```python
from build123d import *

# Parameters (mm, degrees)
IZIM1_R                     = 22.5
Y_KSEKLIK_EKSTR_ZYON1_DEPTH = 32.5
IZIM2_R                     = 17.8
Y_KSEKLIK_EKSTR_ZYON2_DEPTH = 2
RADYUS1_R                   = 0.5
IZIM3_R                     = 13.6
Y_KSEKLIK_EKSTR_ZYON3_DEPTH = 5
RADYUS2_R                   = 2
IZIM4_R                     = 9.05
KES_EKSTR_ZYON1_DEPTH       = 20
RADYUS3_R                   = 0.5
IZIM5_R                     = 18
Y_KSEKLIK_EKSTR_ZYON4_DEPTH = 10.7
IZIM6_R                     = 22.65
Y_KSEKLIK_EKSTR_ZYON5_DEPTH = 5
IZIM7_W                     = 16
IZIM7_H                     = 16
IZIM7_W_2                   = 13
IZIM7_H_2                   = 13
Y_KSEKLIK_EKSTR_ZYON6_DEPTH = 4


with BuildPart() as part:
    # Çizim1 → Yükseklik-Ekstrüzyon1 (new body)
    with BuildSketch(Plane.XY):
        Circle(IZIM1_R)
    extrude(amount=Y_KSEKLIK_EKSTR_ZYON1_DEPTH)

    # Çizim2 → Yükseklik-Ekstrüzyon2 (add)
    with BuildSketch(Plane.XY.offset(32.5)):
        Circle(IZIM2_R)
    extrude(amount=Y_KSEKLIK_EKSTR_ZYON2_DEPTH)

    # Radyus1
    radyus1_edges = [part.edges().sort_by_distance(p)[0] for p in [
        (-17.8, 0, 32.5),
    ]]
    fillet(radyus1_edges, radius=RADYUS1_R)

    # Çizim3 → Yükseklik-Ekstrüzyon3 (add)
    with BuildSketch(Plane.XY.offset(34.5)):
        Circle(IZIM3_R)
    extrude(amount=Y_KSEKLIK_EKSTR_ZYON3_DEPTH)

    # Radyus2
    radyus2_edges = [part.edges().sort_by_distance(p)[0] for p in [
        (-13.6, 0, 34.5),
    ]]
    fillet(radyus2_edges, radius=RADYUS2_R)

    # Çizim4 → Kes-Ekstrüzyon1 (cut)
    with BuildSketch(Plane.XY.offset(39.5)):
        Circle(IZIM4_R)
    extrude(amount=-KES_EKSTR_ZYON1_DEPTH, mode=Mode.SUBTRACT)

    # Radyus3
    radyus3_edges = [part.edges().sort_by_distance(p)[0] for p in [
        (-22.5, 0, 32.5),
    ]]
    fillet(radyus3_edges, radius=RADYUS3_R)

    # Çizim5 → Yükseklik-Ekstrüzyon4 (add)
    with BuildSketch(Plane(origin=(0, 0, 0), x_dir=(-1, 0, 0), z_dir=(0, 0, -1))):
        Circle(IZIM5_R)
    extrude(amount=Y_KSEKLIK_EKSTR_ZYON4_DEPTH)

    # Çizim6 → Yükseklik-Ekstrüzyon5 (add)
    with BuildSketch(Plane(origin=(0, 0, -10.7), x_dir=(-1, 0, 0), z_dir=(0, 0, -1))):
        Circle(IZIM6_R)
    extrude(amount=Y_KSEKLIK_EKSTR_ZYON5_DEPTH)

    # Çizim7 → Yükseklik-Ekstrüzyon6 (add)
    with BuildSketch(Plane(origin=(0, 0, -15.7), x_dir=(-1, 0, 0), z_dir=(0, 0, -1))):
        Rectangle(IZIM7_W, IZIM7_H)
        Rectangle(IZIM7_W_2, IZIM7_H_2, mode=Mode.SUBTRACT)
    extrude(amount=Y_KSEKLIK_EKSTR_ZYON6_DEPTH)


solid = part.part
```
The model under review builds one solid part; all positions refer to its coordinate system, in mm. A direction names the side the tool comes from. Give positions to 0.01 mm unless a question says otherwise; leave off trailing zeros. Write each loop counter-clockwise with the first axis right and the second up, starting at its lowest first coordinate (ties: lowest second). Pieces come first, ordered by that corner, then holes. Notation, with made-up numbers: (-22, -40) -> (-7, -40) arc R34 cw to (-7, -2) -> close; hole circle Ø7 at (-21, 6). An arc over 180 degrees is marked (long way). Answer in a Markdown table with one row per item.
1) Clearance check with flat-ended pins moving along their axes: P1, Ø3, axis at x = -2, z = -17, coming from the -Y side; P2, Ø21, axis at x = 0, y = 0, coming from the +Z side; P3, Ø3, axis at y = -9, z = -4.5, coming from the -X side; P4, Ø4, axis at x = -2, y = -2, coming from the -Z side. State where each tip first meets the part, or that it passes through.
Worked answers:
| item | result |
|---|---|
| P1 | y = -22.62 |
| P2 | z = 39.5 |
| P3 | x = -16.36 |
| P4 | z = -15.7 |
2) Mouldability with a two-part tool opening along Y and no side actions: class faces 1 (the flat face through (-18, -5, 32.5)), 2 (the cylindrical face through (-2.948, -13.277, 37.979)), 3 (the flat face through (6.5, 0, -18)) as +Y half, -Y half, draft (parallel to the pull), parting line (faces both ways), or undercut.
Worked answers:
| item | result |
|---|---|
| face 1 | draft |
| face 2 | parting line |
| face 3 | undercut |
3) For L1, parallel to Z at x = 7, y = 17.5; L2, parallel to Y at x = 0, z = 34; L3, parallel to Y at x = 0, z = 30.25, list the stretches that pass through material, from the lowest coordinate up. Write a range as [from, to].
Worked answers:
| item | result |
|---|---|
| L1 | [-15.7, -10.7], [0, 32.5] |
| L2 | [-17.8, -9.05], [9.05, 17.8] |
| L3 | [-22.5, -9.05], [9.05, 22.5] |
4) Add section A-A on z = 8.5. State the section outline as (x, y) points, plus the area to 3 significant figures.
Worked answers:
| item | result |
|---|---|
| outline | circle Ø45 at (0, 0) |
| area | 1,590 mm² |
5) Tool access review of faces 4 (the cylindrical face through (-3.859, -17.377, 33.74)), 5 (the flat face through (8, 0, -18)), 6 (the flat face through (-7, 17, -10.7)): name each direction out of +Z, -Z, +X, -X, +Y, -Y from which nothing blocks a thin tool from reaching the whole face with its end or side.
Worked answers:
| item | result |
|---|---|
| face 4 | +Z |
| face 5 | -Z, +X, +Y, -Y |
| face 6 | none |
